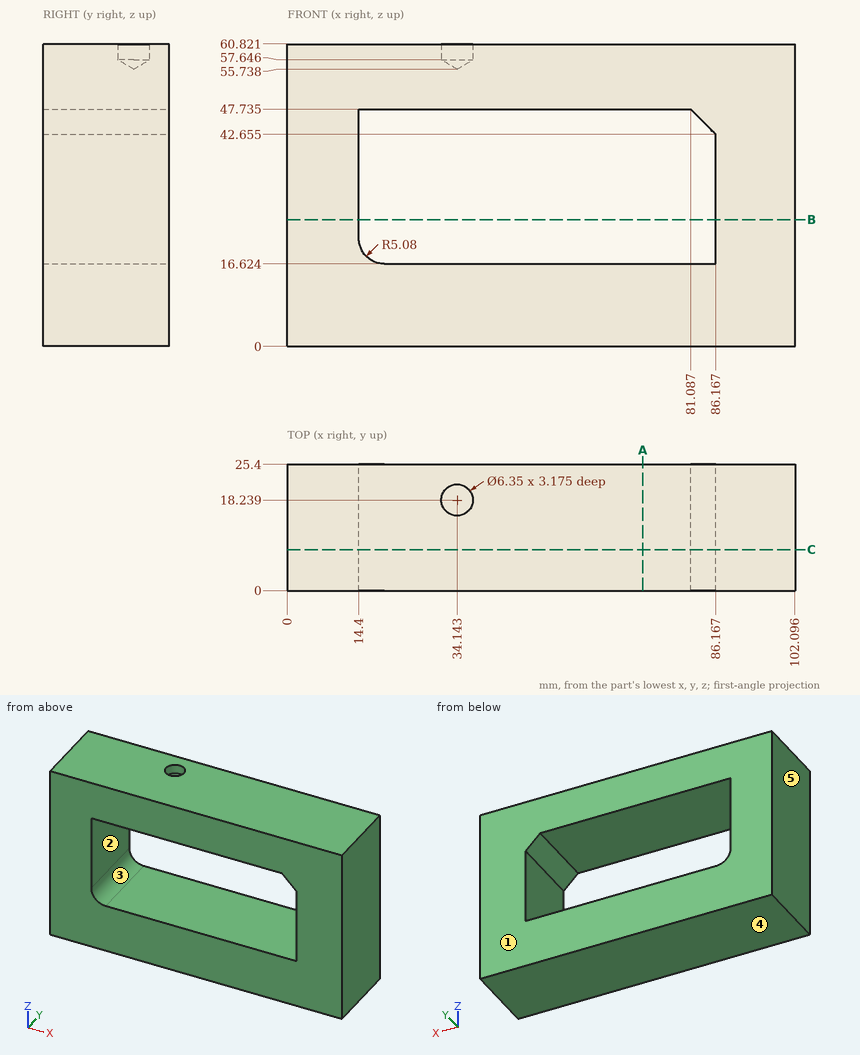
Design review of the part shown in the three views and the two pictorial views. Dimensions are in mm from the part's minimum x, y and z. A direction names the side the tool comes from. Round coordinates to 2 decimals unless told otherwise and drop trailing zeros. Write each loop counter-clockwise with the first axis right and the second up, starting at its lowest first coordinate (ties: lowest second). Pieces come first, ordered by that corner, then holes. Notation, with made-up numbers: M 70,39.5 L 119,39.5 A29 ccw 119,59.5 Z; hole C 57.5,-0.5 d10. An arc over 180 degrees is marked long. Use a Markdown table: item, result. Add a question column.
Q1. We need section A-A, the plane x = 71.5. State the section outline as (y, z) points (1 decimal).
Q2. Insertion check: pin 1 (5 mm diameter, centred on x = 25.5, z = 44.5, fed in from -Y); pin 2 (5.5 mm diameter, centred on x = 34.14, y = 18.24, fed in from +Z). Each pin has a flat end and moves straight along its axis. Give the tip position at first contact, or say it passes through.
Q3. Machinability: for the marked faces 1 and 2, which of the approach directions +Z, -Z, +X, -X, +Y, -Y give a long, thin tool a straight path to every point of the face, cutting with its end or side? Answer none if there is none.
Q4. We need section C-C, the plane y = 8.25. State the section outline as (x, z) points (1 decimal).
Q5. We need section B-B, the plane z = 25.5. State the section outline as (x, y) points, plus the area to 3 significant figures.
Q6. The part is to be moulded in two halves that separate along Z. For the marked faces 3, 4 and 5, say which applies: pulls with the +Z half, pulls with the -Z half, needs draft (parallel to the pull), parting line crosses it, or undercut.
Q7. To check wall thickness, follow line 1 (Z direction, x = 45, y = 12) (1 decimal); line 2 (X direction, y = 9.75, z = 30); line 3 (Z direction, x = 16, y = 2) (1 decimal). State the ranges of each line that lie inside material, in increasing order.
Findings below:
| question | item | result |
|---|---|---|
| 1 | outline | M 0,0 L 25.4,0 L 25.4,16.6 L 0,16.6 Z; M 0,47.7 L 25.4,47.7 L 25.4,60.8 L 0,60.8 Z |
| 2 | pin 1 | passes through |
| 2 | pin 2 | stops at z = 57.39 |
| 3 | face 1 | +Z, -Z, +X, -X, +Y |
| 3 | face 2 | +Y, -Y |
| 4 | outline | M 0,0 L 102.1,0 L 102.1,60.8 L 0,60.8 Z; hole M 14.4,21.7 A5.1 ccw 19.5,16.6 L 86.2,16.6 L 86.2,42.7 L 81.1,47.7 L 14.4,47.7 Z |
| 5 | outline | M 0,0 L 14.4,0 L 14.4,25.4 L 0,25.4 Z; M 86.17,0 L 102.1,0 L 102.1,25.4 L 86.17,25.4 Z |
| 5 | area | 770 mm² |
| 6 | face 3 | undercut |
| 6 | face 4 | pulls with the -Z half |
| 6 | face 5 | needs draft |
| 7 | line 1 | z = 0 to 16.6, 47.7 to 60.8 |
| 7 | line 2 | x = 0 to 14.4, 86.17 to 102.1 |
| 7 | line 3 | z = 0 to 18, 47.7 to 60.8 |
